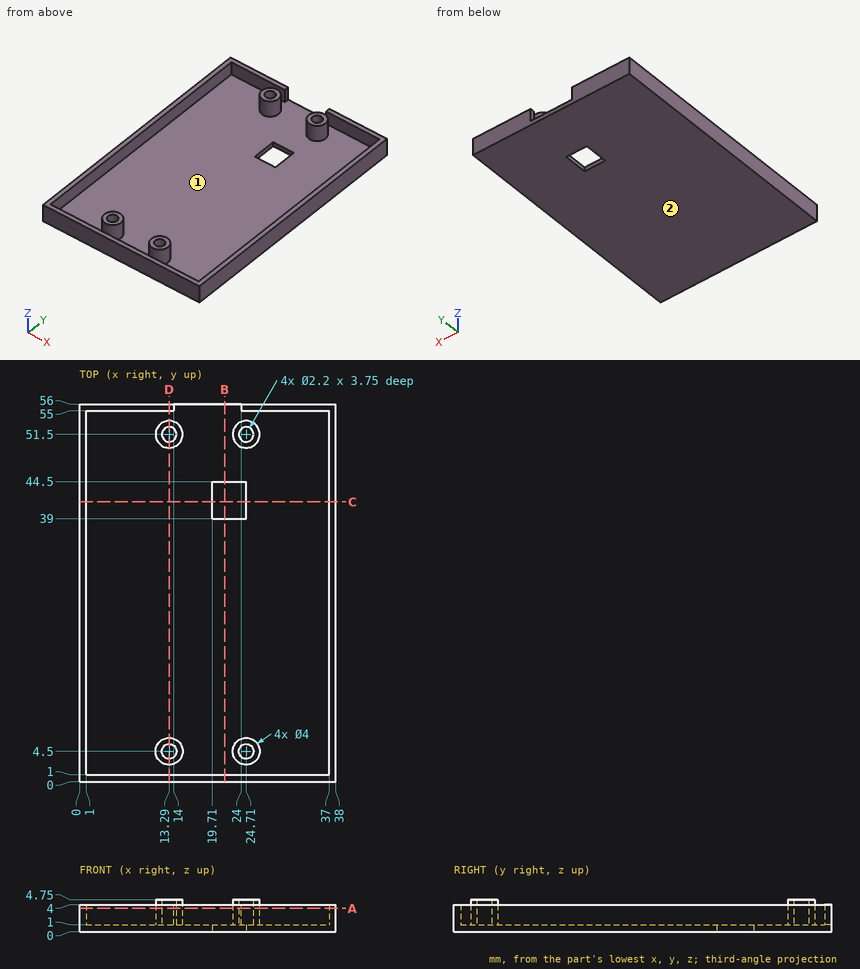
Job drawing, mm, ordinate dimensions from the low corner. One solid piece. Give positions to 0.01 mm unless a question says otherwise; leave off trailing zeros. Loops run counter-clockwise (first coordinate to the right, second up) from the corner with the lowest first, then second, coordinate; pieces in that order, holes last. Notation, with made-up numbers: (65, 19) -> (81, 19) arc R38 ccw to (81, 57) -> close; hole circle Ø3 at (-9.75, 62.25). An arc over 180 degrees is marked (long way). Use a Markdown table: item, result. Add a question column.
(1) Slice it at D-D on x = 13.29. List the corners of the cut face in (y, z), and give its area (3 significant figures).
(2) Wall check: line 1 along Y through (x, z) = (24.71, 3.1); line 2 along X through (y, z) = (4.5, 3.4); line 3 along X through (y, z) = (9, 2.4). Give the ranges that are in metal, low to high.
(3) Slice it at B-B on x = 21.5. List the corners of the cut face in (y, z), and give its area (3 significant figures).
(4) Drop a flat-ended pin along its axis: pin 1 Ø11 at (x, y) = (28, 41.5) entering from +Z. Give the stop position or say it passes through.
(5) Slice it at A-A on z = 3.45. Give the number of separate pieces and of enclosed holes in the cut face, and give its area (3 significant figures).
(6) Mould opens along X. For the marked faces 1 and 2 say: +X half, -X half, draft (parallel to the pull), parting line (faces both ways), or undercut.
(7) Slice it at C-C on y = 41.5. List the corners of the cut face in (x, z).
Filled sheet:
| question | item | result |
|---|---|---|
| 1 | outline | (0, 0) -> (56, 0) -> (56, 4) -> (55, 4) -> (55, 1) -> (53.5, 1) -> (53.5, 4.75) -> (52.6, 4.75) -> (52.6, 1) -> (50.4, 1) -> (50.4, 4.75) -> (49.5, 4.75) -> (49.5, 1) -> (6.5, 1) -> (6.5, 4.75) -> (5.6, 4.75) -> (5.6, 1) -> (3.4, 1) -> (3.4, 4.75) -> (2.5, 4.75) -> (2.5, 1) -> (1, 1) -> (1, 4) -> (0, 4) -> close |
| 1 | area | 75.5 mm2 |
| 2 | line 1 | 0 to 1, 2.5 to 3.4, 5.6 to 6.5, 49.5 to 50.4, 52.6 to 53.5, 55 to 56 |
| 2 | line 2 | 0 to 1, 11.29 to 12.19, 14.39 to 15.29, 22.71 to 23.61, 25.81 to 26.71, 37 to 38 |
| 2 | line 3 | 0 to 1, 37 to 38 |
| 3 | outline | (0, 0) -> (39, 0) -> (39, 1) -> (1, 1) -> (1, 4) -> (0, 4) -> close; (44.5, 0) -> (56, 0) -> (56, 1) -> (44.5, 1) -> close |
| 3 | area | 53.5 mm2 |
| 4 | pin 1 | z = 1 |
| 5 | separate pieces | 5 |
| 5 | enclosed holes | 4 |
| 5 | area | 209 mm2 |
| 6 | face 1 | undercut |
| 6 | face 2 | draft |
| 7 | outline | (0, 0) -> (19.71, 0) -> (19.71, 1) -> (1, 1) -> (1, 4) -> (0, 4) -> close; (24.71, 0) -> (38, 0) -> (38, 4) -> (37, 4) -> (37, 1) -> (24.71, 1) -> close |
